```python
from build123d import *

# Parameters (mm, degrees)
BOSS_EXTRUDE1_DEPTH    = 19.05
SKETCH2_R              = 1.27
CUT_EXTRUDE1_DEPTH     = 50.92377848
F_10_CLEARANCE_HOLE1_D = 5.6134


with BuildPart() as part:
    # Sketch1 → Boss-Extrude1 (new body)
    with BuildSketch(Plane(origin=(0, 0, 0), x_dir=(1, 0, 0), z_dir=(0, 1, 0))):
        with BuildLine():
            Line((39.563039866, -1.582615385), (39.563039866, -25.3365))
            Line((39.563039866, -25.3365), (-39.563039866, -25.3365))
            Line((-39.563039866, -25.3365), (-39.563039866, -1.582615385))
            Line((-39.563039866, -1.582615385), (-20.513039866, -1.582615385))
            ThreePointArc((-20.513039866, -1.582615385), (0, -20.574), (20.513039866, -1.582615385))
            Line((20.513039866, -1.582615385), (39.563039866, -1.582615385))
        make_face()
    extrude(amount=BOSS_EXTRUDE1_DEPTH)

    # Sketch2 → Cut-Extrude1 (cut, through all)
    with BuildSketch(Plane.XY.offset(25.3365)):
        with Locations((33.213039866, 9.525)):
            Circle(SKETCH2_R)
        with Locations((-33.213039866, 9.525)):
            Circle(SKETCH2_R)
    extrude(amount=-CUT_EXTRUDE1_DEPTH, mode=Mode.SUBTRACT)

    # #10 Clearance Hole1 (through all)
    with Locations(Plane.XY.offset(25.3365)):
        with Locations((-33.213039866, 9.525), (33.213039866, 9.525)):
            Hole(F_10_CLEARANCE_HOLE1_D / 2)


solid = part.part
```
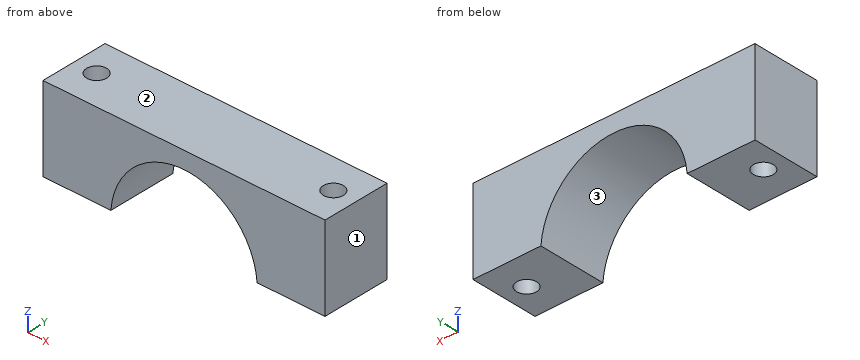
Here's how the part is built. I have some questions about the finished solid (model axes, mm). Face numbers are marked on the shaded views. Coordinates: 2 decimals unless noted, no trailing zeros. Write each loop counter-clockwise with the first axis right and the second up, starting at its lowest first coordinate (ties: lowest second). Pieces come first, ordered by that corner, then holes. Notation, with made-up numbers: (-28, 61.25) - (15, 61.25) arc R30 cw to (15, 84.25) - close; hole circle Ø10 at (34, 25.25). An arc over 180 degrees is marked (long way). One line per item, written item: value.
1) Suppose I cut it at C-C on y = 2.75. Write out the boundary of the cut face in (x, z).
Model answer:
outline: (-39.56, 1.58) - (-20.51, 1.58) arc R20.57 cw to (20.51, 1.58) - (39.56, 1.58) - (39.56, 25.34) - (-39.56, 25.34) - close
2) Suppose I cut it at B-B on x = 33.5. Write out the boundary of the cut face in (y, z).
Model answer:
outline: (0, 1.58) - (6.73, 1.58) - (6.73, 25.34) - (0, 25.34) - close; (12.32, 1.58) - (19.05, 1.58) - (19.05, 25.34) - (12.32, 25.34) - close
3) I need wall thicknesses on line 1 along X through (y, z) = (7, 13); line 2 along X through (y, z) = (9.5, 19); line 3 along X through (y, z) = (18, 11). Which ranges of each line are inside material? Lowest first, please.
Model answer:
line 1: x = -39.56 to -34.44, -31.99 to -15.95, 15.95 to 31.99, 34.44 to 39.56
line 2: x = -39.56 to -36.02, -30.41 to -7.89, 7.89 to 30.41, 36.02 to 39.56
line 3: x = -39.56 to -17.39, 17.39 to 39.56
4) Suppose I cut it at A-A on z = 15.5. Write out the boundary of the cut face in (x, y) (3 decimals).
Model answer:
outline: (-39.563, 0) - (-13.529, 0) - (-13.529, 19.05) - (-39.563, 19.05) - close; (13.529, 0) - (39.563, 0) - (39.563, 19.05) - (13.529, 19.05) - close; hole circle Ø5.613 at (-33.213, 9.525); hole circle Ø5.613 at (33.213, 9.525)
5) Suppose I cut it at D-D on z = 11. Write out the boundary of the cut face in (x, y) (3 decimals), and give its area (3 significant figures).
Model answer:
outline: (-39.563, 0) - (-17.386, 0) - (-17.386, 19.05) - (-39.563, 19.05) - close; (17.386, 0) - (39.563, 0) - (39.563, 19.05) - (17.386, 19.05) - close; hole circle Ø5.613 at (-33.213, 9.525); hole circle Ø5.613 at (33.213, 9.525)
area: 795 mm²
6) We'd pull the mould along X, two halves only. Please class the marked faces 1, 2 and 3: pulls with the +X half, pulls with the -X half, needs draft (parallel to the pull), parting line crosses it, or undercut.
Model answer:
face 1: pulls with the +X half
face 2: needs draft
face 3: undercut
